The figure shows three views and two pictorial views of one solid part (mm, origin at its lowest corner). Answer the questions. Coordinates: 2 decimals unless noted, no trailing zeros. Loops run counter-clockwise (first coordinate to the right, second up) from the corner with the lowest first, then second, coordinate; pieces in that order, holes last. Notation, with made-up numbers: (62, 65) -> (80, 65) arc R25 cw to (80, 96) -> close; hole circle Ø1 at (85, 54.25). An arc over 180 degrees is marked (long way). Answer in a Markdown table with one row per item.
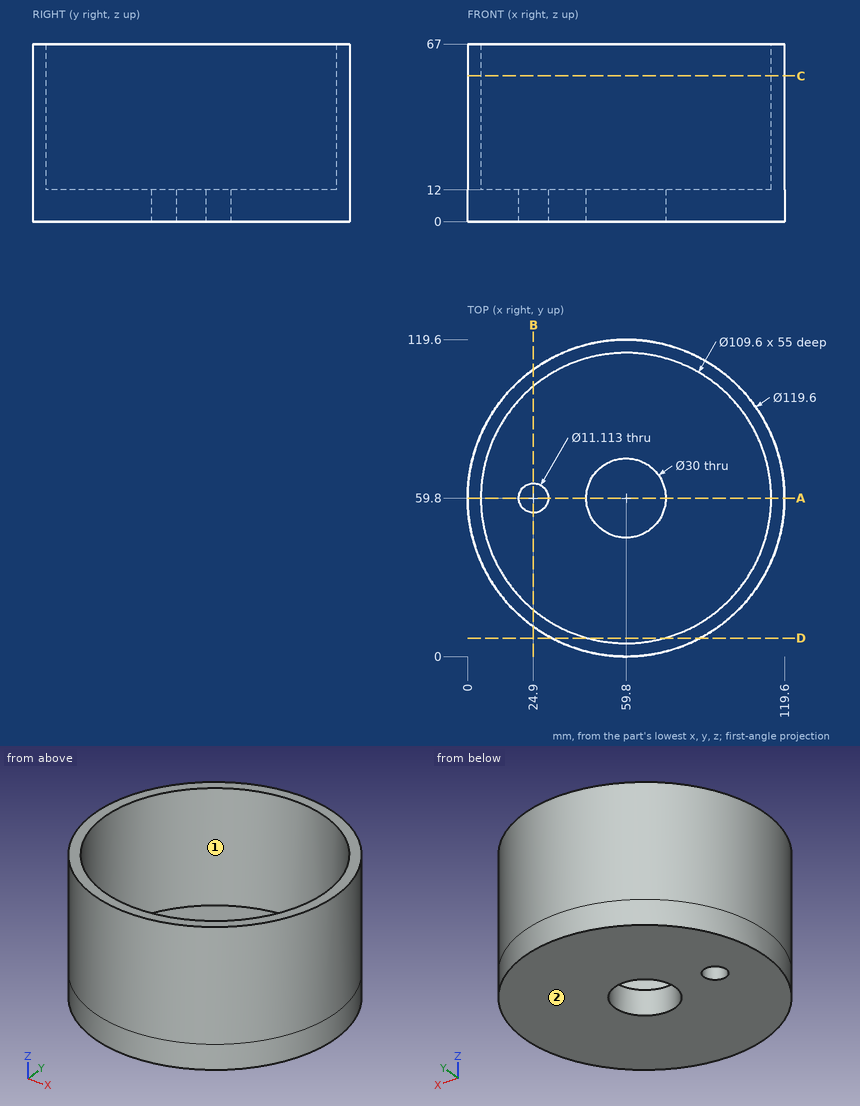
Item 1: A cutting plane is placed at D-D, the plane y = 7. Determine the outline of the cut face in (x, z) (1 decimal).
Findings below:
| item | result |
|---|---|
| outline | (31.7, 0) -> (87.9, 0) -> (87.9, 67) -> (74.5, 67) -> (74.5, 12) -> (45.1, 12) -> (45.1, 67) -> (31.7, 67) -> close |
Item 2: Determine the mould class of the marked faces 1 and 2 for opening direction Y: +Y half, -Y half, draft (parallel to the pull), parting line (faces both ways), or undercut.
Findings below:
| item | result |
|---|---|
| face 1 | undercut |
| face 2 | draft |
Item 3: A cutting plane is placed at C-C, the plane z = 55. Determine the outline of the cut face in (x, y).
Findings below:
| item | result |
|---|---|
| outline | circle Ø119.6 at (59.8, 59.8); hole circle Ø109.6 at (59.8, 59.8) |
Item 4: Find the intervals of material crossed by probe 1 along Y at (x, z) = (59, 5) (1 decimal); probe 2 along X at (y, z) = (59, 6) (1 decimal); probe 3 along X at (y, z) = (62, 4), in increasing order.
Findings below:
| item | result |
|---|---|
| probe 1 | y = 0 to 44.8, 74.8 to 119.6 |
| probe 2 | x = 0 to 19.4, 30.4 to 44.8, 74.8 to 119.6 |
| probe 3 | x = 0.04 to 19.8, 30 to 44.96, 74.64 to 119.56 |
Item 5: A cutting plane is placed at B-B, the plane x = 24.9. Determine the outline of the cut face in (y, z), plus the area to 3 significant figures.
Findings below:
| item | result |
|---|---|
| outline | (11.24, 0) -> (54.24, 0) -> (54.24, 12) -> (17.55, 12) -> (17.55, 67) -> (11.24, 67) -> close; (65.36, 0) -> (108.36, 0) -> (108.36, 67) -> (102.05, 67) -> (102.05, 12) -> (65.36, 12) -> close |
| area | 1,730 mm2 |
Item 6: Flat-ended cylindrical pins translate along their axes: pin 1 Ø2 at (x, z) = (102.5, 31) entering from +Y; pin 2 Ø5 at (y, z) = (88.5, 49) entering from +X (1 decimal); pin 3 Ø8 at (x, z) = (40.5, 26.5) entering from -Y. Find the tip coordinate at first contact, or state that the pin passes through.
Findings below:
| item | result |
|---|---|
| pin 1 | stops at y = 102.66 |
| pin 2 | stops at x = 113.6 |
| pin 3 | stops at y = 1.99 |
Item 7: A cutting plane is placed at A-A, the plane y = 59.8. Determine the outline of the cut face in (x, z), plus the area to 3 significant figures.
Findings below:
| item | result |
|---|---|
| outline | (0, 0) -> (19.34, 0) -> (19.34, 12) -> (5, 12) -> (5, 67) -> (0, 67) -> close; (30.46, 0) -> (44.8, 0) -> (44.8, 12) -> (30.46, 12) -> close; (74.8, 0) -> (119.6, 0) -> (119.6, 67) -> (114.6, 67) -> (114.6, 12) -> (74.8, 12) -> close |
| area | 1,490 mm2 |
